from build123d import *

# Parameters (mm, degrees)
SZKIC1_R                    = 5
SZKIC1_R_2                  = 3
DODANIE_WYCI_GNI_CIE1_DEPTH = 30
SZKIC1_3_R                  = 3
WYTNIJ_WYCI_GNI_CIE1_DEPTH  = 20
ZAOKR_GLENIE1_R             = 5
DODANIE_WYCI_GNI_CIE2_DEPTH = 25


with BuildPart() as part:
    # Szkic1 → Dodanie-wyci_gni_cie1 (new body)
    # profile 1 of 2: a face of its own
    with BuildSketch(Plane.XY):
        Circle(SZKIC1_R)
        Circle(SZKIC1_R_2, mode=Mode.SUBTRACT)
    # profile 2 of 2: a face of its own
    with BuildSketch(Plane.XY):
        Circle(SZKIC1_R_2)
    extrude(amount=DODANIE_WYCI_GNI_CIE1_DEPTH)

    # Szkic1_3 → Wytnij-wyci_gni_cie1 (cut)
    with BuildSketch(Plane.XY):
        Circle(SZKIC1_3_R)
    extrude(amount=WYTNIJ_WYCI_GNI_CIE1_DEPTH, mode=Mode.SUBTRACT)

    # Zaokr_glenie1
    zaokr_glenie1_edges = [part.edges().sort_by_distance(p)[0] for p in [
        (-5, 0, 30),
    ]]
    fillet(zaokr_glenie1_edges, radius=ZAOKR_GLENIE1_R)

    # Szkic4 → Dodanie-wyci_gni_cie2 (add)
    with BuildSketch(Plane(origin=(0, 0, 0), x_dir=(-1, 0, 0), z_dir=(0, 0, -1))):
        with BuildLine():
            ThreePointArc((2.5, -4.330127019), (0, -5), (-2.5, -4.330127019))
            Line((-2.5, -4.330127019), (-2.5, -6.830127019))
            Line((-2.5, -6.830127019), (2.5, -6.830127019))
            Line((2.5, -6.830127019), (2.5, -4.330127019))
        make_face()
    extrude(amount=-DODANIE_WYCI_GNI_CIE2_DEPTH)


solid = part.part
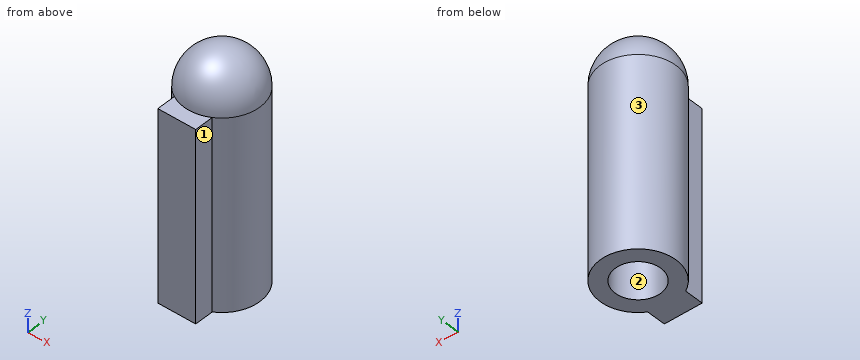
Verification items for the finished model (mm, model axes). Face numbers are marked on the shaded views. Give positions to 0.01 mm unless a question says otherwise; leave off trailing zeros. Write each loop counter-clockwise with the first axis right and the second up, starting at its lowest first coordinate (ties: lowest second). Pieces come first, ordered by that corner, then holes.
(1) Cross-section at D-D (y = 1.75). Enter the section's corners in (x, z), plus the area to 3 significant figures.
(2) Material ranges on line 1 (Y direction, x = 0, z = 4.75); line 2 (X direction, y = -4.75, z = 8); line 3 (Z direction, x = 0.75, y = -5), recorded low to high.
(3) Gauge pin test, flat ends, axial feed: pin 1 (5.5 mm diameter, centred on x = 0, y = 0, fed in from -Z); pin 2 (0.8 mm diameter, centred on y = -5.5, z = 10, fed in from -X); pin 3 (3 mm diameter, centred on x = -3.5, y = 1.5, fed in from +Z); pin 4 (3 mm diameter, centred on x = 1, y = 1.5, fed in from -Z). Record the tip position at first contact, or that the pin passes through.
(4) Cross-section at A-A (x = 0). Enter the section's corners in (y, z), plus the area to 3 significant figures.
(5) Mould release check, pull along X, two halves, no side actions. Record for the marked faces 1, 2 and 3: +X half, -X half, draft (parallel to the pull), parting line (faces both ways), or undercut.
(6) Cross-section at C-C (z = 10.5). Enter the section's corners in (x, y).
(7) Cross-section at B-B (y = 0). Enter the section's corners in (x, z), plus the area to 3 significant figures.
Worked out:
1. outline: (-4.68, 0) - (-2.44, 0) - (-2.44, 20) - (2.44, 20) - (2.44, 0) - (4.68, 0) - (4.68, 25) arc R4.68 ccw to (-4.68, 25) - close
1. area: 171 mm2
2. line 1: y = -6.83 to -3, 3 to 5
2. line 2: x = -2.5 to 2.5
2. line 3: z = 0 to 25
3. pin 1: stops at z = 20
3. pin 2: stops at x = -2.5
3. pin 3: stops at z = 29.44
3. pin 4: stops at z = 0
4. outline: (-6.83, 0) - (-3, 0) - (-3, 20) - (3, 20) - (3, 0) - (5, 0) - (5, 25) arc R5 ccw to (-5, 25) - (-6.83, 25) - close
4. area: 215 mm2
5. face 1: +X half
5. face 2: undercut
5. face 3: parting line
6. outline: (-2.5, -6.83) - (2.5, -6.83) - (2.5, -4.33) arc R5 ccw (long way) to (-2.5, -4.33) - close; hole circle Ø6 at (0, 0)
7. outline: (-5, 0) - (-3, 0) - (-3, 20) - (3, 20) - (3, 0) - (5, 0) - (5, 25) arc R5 ccw to (-5, 25) - close
7. area: 169 mm2
